Check sheet for the modelled part. Datum: model origin and axes. Units: mm. A direction names the side the tool comes from. Give positions to 0.01 mm unless a question says otherwise; leave off trailing zeros. Order: outer loops, then holes, each group sorted by start corner. A loop starts at its lowest first (then second) coordinate and runs counter-clockwise, first axis right, second up.
```python
from build123d import *

# Parameters (mm, degrees)
F1_DEPTH  = 50
F2_T      = -2.5
F3_W      = 5
F3_H      = 6
F3_W_2    = 3
F3_W_3    = 6
F4_DEPTH  = 50
F5_R      = 1.5
F6_DEPTH  = 5
F8_DEPTH  = 5
F10_DEPTH = 6


with BuildPart() as f1:
    # F0 (on Front) → F1 (new body)
    with BuildSketch(Plane.XZ):
        with BuildLine():
            ThreePointArc((0, -45), (24.9125199529, -40.428169894), (45, -25))
            Line((45, -25), (0, -25))
            Line((0, -25), (0, -45))
        make_face()
        with BuildLine():
            Line((0, -25), (45, -25))
            Line((45, -25), (45, 25))
            Line((45, 25), (35, 25))
            Line((35, 25), (35, 5))
            ThreePointArc((35, 5), (17.6776695297, 1.2563132924), (0, 0))
            Line((0, 0), (0, -25))
        make_face()
        with BuildLine():
            Line((0, -45), (0, -25))
            Line((0, -25), (-45, -25))
            ThreePointArc((-45, -25), (-24.9125199529, -40.428169894), (0, -45))
        make_face()
        with BuildLine():
            Line((-45, -25), (0, -25))
            Line((0, -25), (0, 0))
            ThreePointArc((0, 0), (-17.6776695297, 1.2563132924), (-35, 5))
            Line((-35, 5), (-35, 25))
            Line((-35, 25), (-45, 25))
            Line((-45, 25), (-45, -25))
        make_face()
        with BuildLine():
            Line((35, 25), (45, 25))
            Line((45, 25), (45, 35))
            ThreePointArc((45, 35), (42.0710678119, 27.9289321881), (35, 25))
        make_face()
        with BuildLine():
            Line((-45, 35), (-45, 25))
            Line((-45, 25), (-35, 25))
            ThreePointArc((-35, 25), (-42.0710678119, 27.9289321881), (-45, 35))
        make_face()
    extrude(amount=F1_DEPTH)

    # F2
    f2_openings = [f1.faces().sort_by_distance(p)[0] for p in [
        (-24.91252, -25, -40.42817),
        (24.91252, -25, -40.42817),
        (0, 0, -15.155819),
    ]]
    offset(amount=F2_T, openings=f2_openings, kind=Kind.INTERSECTION)

    # F3 (on Front) → F4 (join)
    with BuildSketch(Plane.XZ):
        with Locations((-40, 15.2549841851)):
            Rectangle(F3_W, F3_H)
        with Locations((40, 15.2549841851)):
            Rectangle(F3_W, F3_H)
        with Locations((1.5, -3)):
            Rectangle(F3_W_2, F3_H)
        with Locations((-1.5, -3)):
            Rectangle(F3_W_2, F3_H)
        Polygon((-42.5, -9.7450158149), (-42.5, -12.7450158149), (-42.5, -15.7450158149), (-36.5, -15.7450158149), (-36.5, -9.7450158149), align=None)
        with Locations((39.5, -12.7450158149)):
            Rectangle(F3_W_3, F3_H)
    extrude(amount=F4_DEPTH)

    # F5 (on face) → F6 (join)
    with BuildSketch(Plane.XZ):
        with Locations((-40, 15.2549841851)):
            Circle(F5_R)
        with Locations((-39.5, -12.7450158149)):
            Circle(F5_R)
        with Locations((40, 15.2549841851)):
            Circle(F5_R)
        with Locations((39.5, -12.7450158149)):
            Circle(F5_R)
        with Locations((0, -3)):
            Circle(F5_R)
    extrude(amount=-F6_DEPTH)

    # F7 (on Top) → F8 (join)
    with BuildSketch(Plane.XY):
        with BuildLine():
            Line((9, 0), (-9, 0))
            ThreePointArc((-9, 0), (0, -9.3268755147), (9, 0))
        make_face()
    extrude(amount=F8_DEPTH)

    # F9 (on Top) → F10 (cut)
    with BuildSketch(Plane.XY):
        with BuildLine():
            Line((7.5, 0), (-7.5, 0))
            ThreePointArc((-7.5, 0), (0, -7.5508031077), (7.5, 0))
        make_face()
    extrude(amount=F10_DEPTH, mode=Mode.SUBTRACT)


solid = f1.part
```
(1) Material ranges on L1, parallel to X at y = -24.5, z = 7.5; L2, parallel to X at y = -30, z = -5; L3, parallel to X at y = -33, z = 18, recorded low to high.
Response values:
L1: x = -45 to -42.5, -37.5 to -35, 35 to 37.5, 42.5 to 45
L2: x = -45 to -42.5, -3 to 3, 42.5 to 45
L3: x = -45 to -35, 35 to 45
(2) Gauge pin test, flat ends, axial feed: pin 1 Ø1.5 at (x, y) = (6.5, -4) entering from +Z; pin 2 Ø4 at (x, y) = (-32, -14.5) entering from +Z; pin 3 Ø2 at (x, z) = (14.5, -24.5) entering from +Y; pin 4 Ø19 at (x, z) = (-22, 15) entering from +Y. Record the tip position at first contact, or that the pin passes through.
Response values:
pin 1: stops at z = 5
pin 2: stops at z = 4.71
pin 3: stops at y = -47.5
pin 4: passes through
(3) Release check for a two-part mould opening along X. For faces 1 (the face through (0, 5, -3)), 2 (the face through (-35, -25, 15)) record: released by +X, released by -X, zero draft, split by the parting line, or undercut.
Response values:
face 1: zero draft
face 2: undercut
(4) Cross-section at A-A on z = -8.5. Enter the section's corners in (x, y).
Response values:
outline: (-45, -50) - (45, -50) - (45, 0) - (42.5, 0) - (42.5, -47.5) - (-42.5, -47.5) - (-42.5, 0) - (-45, 0) - close
(5) Cross-section at B-B on y = -12.5. Count the separate pieces of the cut face and the enclosed holes in it, then the cut area to 3 significant figures.
Response values:
separate pieces: 1
enclosed holes: 2
area: 755 mm2
(6) Set-up check for faces 3 (the face through (40, -23, 18.255)), 4 (the face through (0, -8, 5)), 5 (the face through (0, -23, -6)): record each of +Z, -Z, +X, -X, +Y, -Y from which the full face is reachable in a straight line by a thin tool's end or side.
Response values:
face 3: +Y
face 4: +Z, +Y, -Y
face 5: -Z, +Y
(7) Cross-section at C-C on x = -26. Enter the section's corners in (y, z).
Response values:
outline: (-50, -39.93) - (-47.5, -39.93) - (-47.5, 0.18) - (0, 0.18) - (0, 2.73) - (-50, 2.73) - close
